```python
from build123d import *

# Parameters (mm, degrees)
ESQUISSE1_W                     = 42
ESQUISSE1_H                     = 16
BOSS_EXTRU_1_DEPTH              = 41.83
ESQUISSE2_W                     = 22
ESQUISSE2_H                     = 31.83
ENL_V_MAT_EXTRU_1_DEPTH         = 50.464622712
CONG_1_R                        = 5
D_GAGEMENT_M3_51_D              = 3.9
DIAM_TRE_DU_PER_AGE_4_5_4_5_2_D = 4.5
ENL_V_MAT_EXTRU_2_DEPTH         = 17


with BuildPart() as part:
    # Esquisse1 → Boss.-Extru.1 (new body)
    with BuildSketch(Plane.XY):
        Rectangle(ESQUISSE1_W, ESQUISSE1_H)
    extrude(amount=BOSS_EXTRU_1_DEPTH)

    # Esquisse2 → Enlèv. mat.-Extru.1 (cut, through all)
    with BuildSketch(Plane.XZ.offset(8)):
        with Locations((-10, 15.915)):
            Rectangle(ESQUISSE2_W, ESQUISSE2_H)
    extrude(amount=-ENL_V_MAT_EXTRU_1_DEPTH, mode=Mode.SUBTRACT)

    # Congé1
    cong_1_edges = [part.edges().sort_by_distance(p)[0] for p in [
        (-10, 8, 31.83),
        (-21, 0, 31.83),
        (1, 8, 15.915),
        (1, 0, 31.83),
        (1, -8, 15.915),
        (-10, -8, 31.83),
    ]]
    fillet(cong_1_edges, radius=CONG_1_R)

    # Dégagement M3.51 (through all)
    with Locations(Plane(origin=(21, 0, 0), x_dir=(0, 0, -1), z_dir=(1, 0, 0))):
        with Locations((-19.425, 0)):
            Hole(D_GAGEMENT_M3_51_D / 2)

    # Diamètre du perçage Ø4.5 (4.5)2 (through all)
    with Locations(Plane.XY.offset(41.83)):
        with Locations((-16, 0), (-4, 0)):
            Hole(DIAM_TRE_DU_PER_AGE_4_5_4_5_2_D / 2)

    # Esquisse7 → Enlèv. mat.-Extru.2 (cut)
    with BuildSketch(Plane(origin=(1, 0, 0), x_dir=(0, 0, -1), z_dir=(1, 0, 0))):
        Polygon((-24.10153718, 0), (-21.76326859, -4.05), (-17.08673141, -4.05), (-14.74846282, 0), (-17.08673141, 4.05), (-21.76326859, 4.05), align=None)
    extrude(amount=ENL_V_MAT_EXTRU_2_DEPTH, mode=Mode.SUBTRACT)


solid = part.part
```
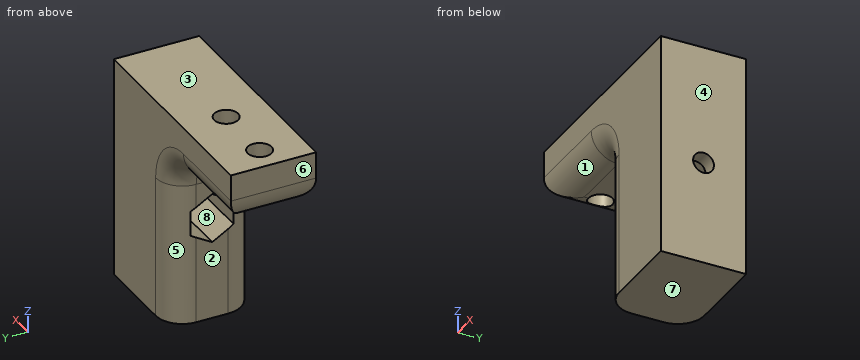
CAD build for the part. Positions are in the model's coordinates, mm. Face numbers are marked on the shaded views. A direction names the side the tool comes from. Coordinates: 2 decimals unless noted, no trailing zeros. Order: outer loops, then holes, each group sorted by start corner. A loop starts at its lowest first (then second) coordinate and runs counter-clockwise, first axis right, second up. Notation, with made-up numbers: M 72.5,8.5 L 82.5,8.5 A9 ccw 82.5,12.5 Z; hole C -37,58 d8. An arc over 180 degrees is marked long. Write each question's results on one line, items separated by ' | '. Start each with the question number.
Q1. Cut at C-C (y = -5). List the corners of the cut face in (x, z).
Q2. Pull direction Z, two halves, no side cores. Call the marked faces 6, 7 and 8: +Z half, -Z half, draft (parallel to the pull), parting line (faces both ways), or undercut.
Q3. Cut at A-A (x = 8). List the corners of the cut face in (y, z).
Q4. Flat gauge pins, fed straight in: P1, Ø6.5, axis at y = -1.5, z = 4.5, coming from the -X side; P2, Ø6.5, axis at y = 0, z = 19.5, coming from the -X side; P3, Ø2, axis at x = -5.5, z = 32.5, coming from the -Y side; P4, Ø2.5, axis at y = 0, z = 19.425, coming from the +X side. Where does each tip first touch, or does it go through?
Q5. Drill centre lines: probe 1 along X at (y, z) = (0, 38.75); probe 2 along Y at (x, z) = (-16, 38.25); probe 3 along X at (y, z) = (-0.5, 6). Where is each one in solid material? Low to high. Write a range as from..to.
Q6. Which spindle directions (+Z, -Z, +X, -X, +Y, -Y) get a long thin tool onto all of the face, cutting with end or side? Do the marked faces 1, 2, 3, 4 and 5. Say none if no direction does.
Q7. Cut at D-D (x = -5). List the corners of the cut face in (y, z).
Q8. Cut at B-B (z = 18). List the corners of the cut face in (x, y), then the cut area to 3 significant figures.
Found:
1) outline: M -21,36.83 A5 ccw -18,32.25 L -4,32.25 A5.42 cw 1.42,26.83 L 1.42,0 L 21,0 L 21,41.83 L -21,41.83 Z
2) face 6: draft | face 7: -Z half | face 8: undercut
3) outline: M -8,0 L 8,0 L 8,41.83 L -8,41.83 Z; hole M -4.05,17.09 L 0,14.75 L 4.05,17.09 L 4.05,21.76 L 0,24.1 L -4.05,21.76 Z
4) P1: x = 1 | P2: x = 18 | P3: y = -6.73 | P4: through
5) probe 1: -21..-18.25, -13.75..-6.25, -1.75..21 | probe 2: -8..-2.25, 2.25..8 | probe 3: 1..21
6) face 1: -Z, -X, -Y | face 2: -Z, -X, +Y, -Y | face 3: +Z, +X, -X, +Y, -Y | face 4: +Z, -Z, +X, +Y, -Y | face 5: -Z, -X, +Y
7) outline: M -8,36.83 A5 ccw -3,31.83 L -2.02,31.83 L -2.02,41.83 L -8,41.83 Z; M 2.02,31.83 L 3,31.83 A5 ccw 8,36.83 L 8,41.83 L 2.02,41.83 Z
8) outline: M 1.11,-4.05 A5 ccw 6,-8 L 21,-8 L 21,-1.33 L 18,-1.33 L 18,-4.05 Z; M 1.11,4.05 L 18,4.05 L 18,1.33 L 21,1.33 L 21,8 L 6,8 A5 ccw Z | area: 164 mm²
